```python
from build123d import *

# Parameters (mm, degrees)
F0_W     = 22.0889396991
F0_H     = 5
F1_DEPTH = 10
F0_W_2   = 2
F0_H_2   = 2
F0_W_3   = 0.7
F2_DEPTH = 4.5
F3_R     = 4.99999
F4_R     = 0.5


# Not quite as in the source:
# - a fillet or chamfer is up to 0.001 mm smaller than in the source, because OpenCascade refuses the exact size


with BuildPart() as f1:
    # F0 (on Top) → F1 (new body)
    with BuildSketch(Plane.XY):
        Polygon((-0.9434188306, 20), (-0.9434188306, 0), (5.6756753474, 0), (5.6756753474, 5), (2.5402316824, 5), (2.5402316824, 15), (5.6756753474, 15), (5.6756753474, 20), align=None)
        Polygon((5.6756753474, 5), (5.6756753474, 0), (39.0565811694, 0), (39.0565811694, 7), (39.0565811694, 9), (39.0565811694, 11), (39.0565811694, 13), (39.0565811694, 20), (32.7646150465, 20), (32.7646150465, 15), (32.7646150465, 5), align=None)
        with Locations((16.720145197, 17.5)):
            Rectangle(F0_W, F0_H)
    extrude(amount=F1_DEPTH)

    # F0 (on Top) → F2 (join)
    with BuildSketch(Plane.XY):
        Polygon((39.0565811694, 9), (39.0565811694, 7), (41.0565811694, 7), (41.0565811694, 9), (39.7565811694, 9), align=None)
        with Locations((42.0565811694, 8)):
            Rectangle(F0_W_2, F0_H_2)
        Polygon((43.0565811694, 7), (41.0565811694, 7), (41.0565811694, 6.25), align=None)
        Polygon((39.0565811694, 13), (39.0565811694, 11), (39.7565811694, 11), (41.0565811694, 11), (41.0565811694, 13), align=None)
        with Locations((42.0565811694, 12)):
            Rectangle(F0_W_2, F0_H_2)
        Polygon((41.0565811694, 13.75), (41.0565811694, 13), (43.0565811694, 13), align=None)
        with Locations((39.4065811694, 10)):
            Rectangle(F0_W_3, F0_H_2)
    extrude(amount=F2_DEPTH)

    # F3 (radius 5 in the source; OpenCascade refuses exactly that, so slightly less here)
    f3_edges = [f1.edges().sort_by_distance(p)[0] for p in [
        (2.540232, 15, 5),
        (2.540232, 5, 5),
        (32.764615, 5, 5),
        (32.764615, 20, 5),
    ]]
    fillet(f3_edges, radius=F3_R)

    # F4
    f4_edges = [f1.edges().sort_by_distance(p)[0] for p in [
        (39.056581, 13, 2.25),
        (39.056581, 7, 2.25),
        (41.056581, 7, 2.25),
        (41.056581, 13, 2.25),
        (39.756581, 11, 2.25),
        (39.756581, 9, 2.25),
    ]]
    fillet(f4_edges, radius=F4_R)


solid = f1.part
```
Model file for the job. Use its own axes, mm. A direction names the side the tool comes from. Give positions to 0.01 mm unless a question says otherwise; leave off trailing zeros. Write each loop counter-clockwise with the first axis right and the second up, starting at its lowest first coordinate (ties: lowest second). Pieces come first, ordered by that corner, then holes. Notation, with made-up numbers: (33.25, -9) - (44.25, -9) arc R11 cw to (44.25, 10) - close; hole circle Ø3 at (89.25, 51). An arc over 180 degrees is marked (long way). One line per question, with ' | ' between items. Start each with the question number.
(1) Slice it at A-A on y = 5.5. Write the cut outline in (x, z), plus the area to 3 significant figures.
(2) Wall check: line 1 along Y through (x, z) = (15.5, 4); line 2 along X through (y, z) = (15.25, 9.25); line 3 along X through (y, z) = (10, 5.25). Give the ranges that are in metal, low to high. Write a range as from..to.
(3) Slice it at B-B on x = 25.5. Write the cut outline in (y, z), plus the area to 3 significant figures.
(4) Pin check, flat tips, straight feed: P1, Ø3, axis at x = 42, y = 9, coming from the +Z side; P2, Ø3, axis at x = 42.5, z = 2.5, coming from the +Y side; P3, Ø0.8, axis at x = 40, z = 2, coming from the -Y side. Stop position of each tip, or through.
(5) Two-plate mould, pull along X, no slides. Class faces 6 (the face through (4.04, 6.43, 5.07)), 7 (the face through (40, 7, 2)), 8 (the face through (42.07, 13.37, 2.22)), 9 (the face through (42, 11, 2)): +X half, -X half, draft (parallel to the pull), parting line (faces both ways), or undercut.
(6) 3-axis set-ups, long thin cutter, end or side, ignore diameter. For faces 1 (the face through (19, 0, 5)), 2 (the face through (3.97, 13.5, 5.07)), 3 (the face through (43.057, 12, 2)), 4 (the face through (31.339, 6.504, 5.07)), 5 (the face through (39.757, 10, 2)): which of +Z, -Z, +X, -X, +Y, -Y reach the whole face in a straight line?
Results below:
1) outline: (-0.94, 0) - (5.36, 0) - (5.36, 10) - (-0.94, 10) - close; (29.94, 0) - (39.06, 0) - (39.06, 10) - (29.94, 10) - close | area: 154 mm^2
2) line 1: 0..5, 15..20 | line 2: -0.94..27.76, 32.77..39.06 | line 3: -0.94..2.54, 32.76..39.06
3) outline: (0, 0) - (5, 0) - (5, 10) - (0, 10) - close; (15, 0) - (20, 0) - (20, 10) - (15, 10) - close | area: 100 mm^2
4) P1: z = 4.5 | P2: y = 13.75 | P3: y = 7
5) face 6: undercut | face 7: undercut | face 8: +X half | face 9: draft
6) face 1: +Z, -Z, +X, -X, -Y | face 2: +Z, -Z | face 3: +Z, -Z, +X, +Y, -Y | face 4: +Z, -Z, +Y | face 5: +Z, -Z, +X
